from build123d import *

# Parameters (mm, degrees)
F0_R     = 1.5
F1_DEPTH = 25
F2_R     = 0.2


with BuildPart() as f1:
    # F0 (on Top) → F1 (new body)
    with BuildSketch(Plane.XY):
        Polygon((3, 1.732051), (0, 3.464102), (-3, 1.732051), (-3, -1.732051), (0, -3.464102), (3, -1.732051), align=None)
        Circle(F0_R, mode=Mode.SUBTRACT)
    extrude(amount=F1_DEPTH)

    # F2
    f2_edges = [f1.edges().sort_by_distance(p)[0] for p in [
        (1.5, 2.598076, 25),
        (-1.5, 2.598076, 25),
        (-3, 0, 25),
        (-1.5, -2.598076, 25),
        (1.5, -2.598076, 25),
        (3, 0, 25),
        (-1.5, 0, 25),
        (1.5, 2.598076, 0),
        (-1.5, 2.598076, 0),
        (-3, 0, 0),
        (-1.5, -2.598076, 0),
        (1.5, -2.598076, 0),
        (3, 0, 0),
        (-1.5, 0, 0),
    ]]
    fillet(f2_edges, radius=F2_R)


solid = f1.part
Read the model definition and answer for the solid it produces. Units are mm, in the model's axes. Round coordinates to 2 decimals unless told otherwise and drop trailing zeros. Write each loop counter-clockwise with the first axis right and the second up, starting at its lowest first coordinate (ties: lowest second). Pieces come first, ordered by that corner, then holes.
1. Determine the mould class of faces 1 (the face through (-1.49, 2.54, 0.06)), 2 (the face through (1.49, -2.54, 0.06)), 3 (the face through (-1.5, 0.07, 12.33)) for opening direction Y: pulls with the +Y half, pulls with the -Y half, needs draft (parallel to the pull), parting line crosses it, or undercut.
2. The part is cut by section A-A, the plane z = 8. Determine the outline of the cut face in (x, y), then the cut area to 3 significant figures.
3. The part is cut by section B-B, the plane y = 0. Determine the outline of the cut face in (x, z).
4. Straight lines are drawn through the part: L1, parallel to Z at x = 1.75, y = -2.25; L2, parallel to X at y = 0.75, z = 3.75; L3, parallel to X at y = -1, z = 9. For each, find the intervals that lie inside material, in ascending order.
Values:
1. face 1: pulls with the +Y half
1. face 2: pulls with the -Y half
1. face 3: undercut
2. outline: (-3, -1.73) - (0, -3.46) - (3, -1.73) - (3, 1.73) - (0, 3.46) - (-3, 1.73) - close; hole circle Ø3 at (0, 0)
2. area: 24.1 mm2
3. outline: (-3, 0.2) arc R0.2 ccw to (-2.8, 0) - (-1.7, 0) arc R0.2 ccw to (-1.5, 0.2) - (-1.5, 24.8) arc R0.2 ccw to (-1.7, 25) - (-2.8, 25) arc R0.2 ccw to (-3, 24.8) - close; (1.5, 0.2) arc R0.2 ccw to (1.7, 0) - (2.8, 0) arc R0.2 ccw to (3, 0.2) - (3, 24.8) arc R0.2 ccw to (2.8, 25) - (1.7, 25) arc R0.2 ccw to (1.5, 24.8) - close
4. L1: z = 0 to 25
4. L2: x = -3 to -1.3, 1.3 to 3
4. L3: x = -3 to -1.12, 1.12 to 3
